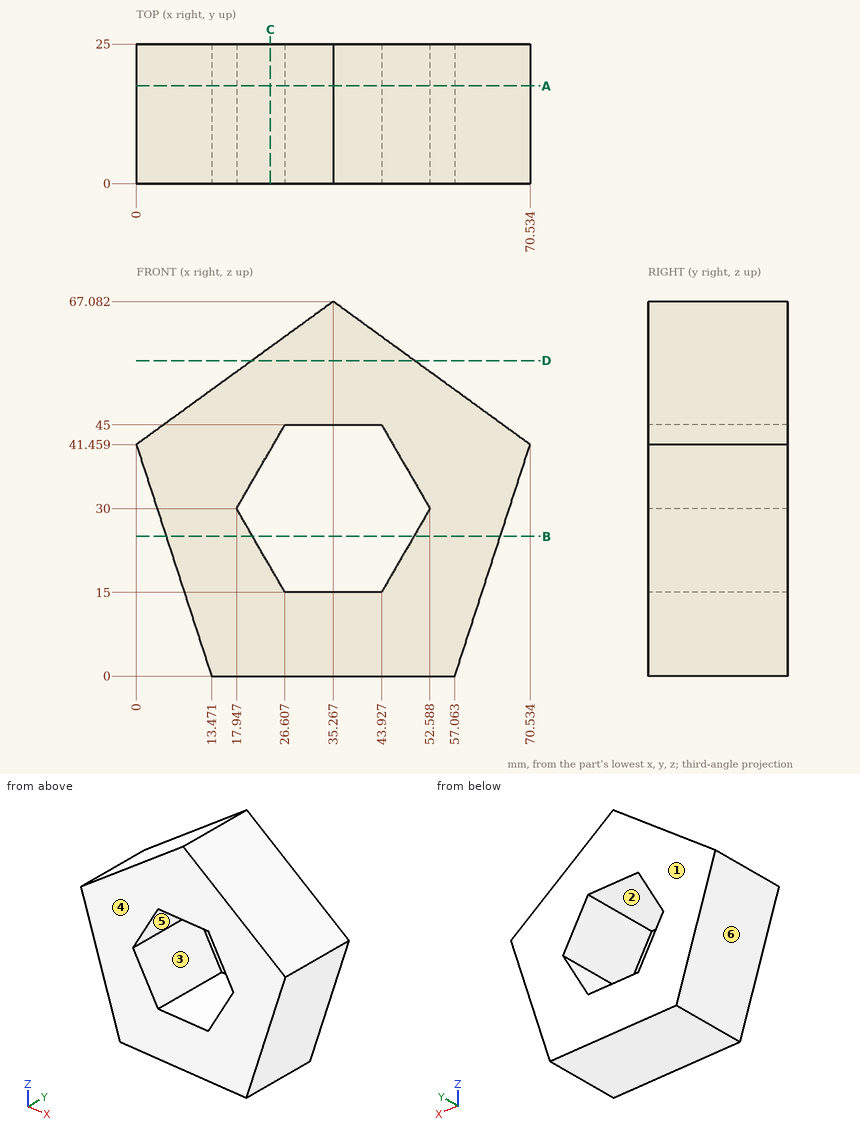
Geometry check sheet. Reference: drawing and pictorial views, mm from the part's lowest x, y, z. A direction names the side the tool comes from. Coordinates: 2 decimals unless noted, no trailing zeros. Loops run counter-clockwise (first coordinate to the right, second up) from the corner with the lowest first, then second, coordinate; pieces in that order, holes last. Notation, with made-up numbers: M 5.25,23.25 L 60.25,23.25 A19 ccw 60.25,34.25 Z; hole C 27,3 d6. An arc over 180 degrees is marked long. One line per item, written item: value.
1. Section check A-A on y = 17.5. Record the cut outline in (x, z) (1 decimal), plus the area to 3 significant figures.
Answers follow:
outline: M 0,41.5 L 13.5,0 L 57.1,0 L 70.5,41.5 L 35.3,67.1 Z; hole M 17.9,30 L 26.6,15 L 43.9,15 L 52.6,30 L 43.9,45 L 26.6,45 Z
area: 2,490 mm^2
2. Mould release check, pull along X, two halves, no side actions. Record for the marked faces 3, 4, 5 and 6: pulls with the +X half, pulls with the -X half, needs draft (parallel to the pull), parting line crosses it, or undercut.
Answers follow:
face 3: undercut
face 4: needs draft
face 5: undercut
face 6: pulls with the -X half
3. Section check C-C on x = 24. Record the cut outline in (y, z) (1 decimal), plus the area to 3 significant figures.
Answers follow:
outline: M 0,0 L 25,0 L 25,19.5 L 0,19.5 Z; M 0,40.5 L 25,40.5 L 25,58.9 L 0,58.9 Z
area: 948 mm^2
4. Section check D-D on z = 56.5. Record the cut outline in (x, y), plus the area to 3 significant figures.
Answers follow:
outline: M 20.7,0 L 49.83,0 L 49.83,25 L 20.7,25 Z
area: 728 mm^2
5. Section check B-B on z = 25. Record the cut outline in (x, y).
Answers follow:
outline: M 5.35,0 L 20.83,0 L 20.83,25 L 5.35,25 Z; M 49.7,0 L 65.19,0 L 65.19,25 L 49.7,25 Z
6. Gauge pin test, flat ends, axial feed: P1, Ø4, axis at y = 15.5, z = 53, coming from the +X side; P2, Ø6, axis at y = 8.5, z = 14, coming from the +X side; P3, Ø12, axis at x = 50.5, y = 6.5, coming from the +Z side (1 decimal). Record the tip position at first contact, or that the pin passes through.
Answers follow:
P1: x = 57.4
P2: x = 62.59
P3: z = 60.4
7. Material ranges on line 1 along Z through (x, y) = (30, 16.5) (1 decimal); line 2 along Z through (x, y) = (22, 7.5) (1 decimal); line 3 along X through (y, z) = (5.5, 27.5) (1 decimal), recorded low to high. Write a range as from..to.
Answers follow:
line 1: 0..15, 45..63.3
line 2: 0..23, 37..57.4
line 3: 4.5..19.4, 51.1..66
8. Set-up check for the marked faces 1 and 2: record each of +Z, -Z, +X, -X, +Y, -Y from which the full face is reachable in a straight line by a thin tool's end or side.
Answers follow:
face 1: +Z, -Z, +X, -X, +Y
face 2: +Y, -Y
